For this review, take the finished solid that the model builds, in its own axes (mm). A direction names the side the tool comes from. Give positions to 0.01 mm unless a question says otherwise; leave off trailing zeros. Order: outer loops, then holes, each group sorted by start corner. A loop starts at its lowest first (then second) coordinate and runs counter-clockwise, first axis right, second up.
from build123d import *

# Parameters (mm, degrees)
SKETCH_1_R      = 2.5
EXTRUDE_1_DEPTH = 3
THICKEN_1_DEPTH = 2
FILLET_6_R      = 4


# Read off the part's stored shape, not the designer's step: 加厚1
with BuildPart() as part:
    # 草图1 → 凸台-拉伸1 (new body)
    with BuildSketch(Plane.XZ):
        with BuildLine():
            Line((-97.488460856, 0), (-69, 0))
            ThreePointArc((-69, 0), (-65, -4), (-61, 0))
            Line((-61, 0), (61, 0))
            ThreePointArc((61, 0), (65, -4), (69, 0))
            Line((69, 0), (97.488460856, 0))
            ThreePointArc((97.488460856, 0), (79.00867922, -47.979553361), (38.781438859, -80))
            Line((38.781438859, -80), (15.564382416, -80))
            ThreePointArc((15.564382416, -80), (0, -70.5), (-15.564382416, -80))
            Line((-15.564382416, -80), (-38.781438859, -80))
            ThreePointArc((-38.781438859, -80), (-79.00867922, -47.979553361), (-97.488460856, 0))
        make_face()
        with Locations(Location((75, -15, 0), (0, 0, 270))):
            Circle(SKETCH_1_R, mode=Mode.SUBTRACT)
    extrude(amount=EXTRUDE_1_DEPTH)

    # 加厚1 outline → 加厚1 (add)
    with BuildSketch(Plane(origin=(0, 0, 0), x_dir=(1, 0, 0), z_dir=(0, 1, 0))):
        with BuildLine():
            ThreePointArc((16.853782958, 77.8), (0, 68.3), (-16.853782958, 77.8))
            Line((-16.853782958, 77.8), (-38.324926614, 77.8))
            ThreePointArc((-38.324926614, 77.8), (-76.642398339, 47.476802076), (-95.019997895, 2.2))
            Line((-95.019997895, 2.2), (-70.796550698, 2.2))
            ThreePointArc((-70.796550698, 2.2), (-65, 6.2), (-59.203449302, 2.2))
            Line((-59.203449302, 2.2), (59.203449302, 2.2))
            ThreePointArc((59.203449302, 2.2), (65, 6.2), (70.796550698, 2.2))
            Line((70.796550698, 2.2), (95.019997895, 2.2))
            ThreePointArc((95.019997895, 2.2), (76.642398339, 47.476802076), (38.324926614, 77.8))
            Line((38.324926614, 77.8), (16.853782958, 77.8))
        make_face()
        with BuildLine():
            Line((-38.115613599, 76.8), (-17.408331339, 76.8))
            ThreePointArc((-17.408331339, 76.8), (0, 67.3), (17.408331339, 76.8))
            Line((17.408331339, 76.8), (38.115613599, 76.8))
            ThreePointArc((38.115613599, 76.8), (75.562692375, 47.247877874), (93.876514635, 3.2))
            Line((93.876514635, 3.2), (71.449806199, 3.2))
            ThreePointArc((71.449806199, 3.2), (65, 7.2), (58.550193801, 3.2))
            Line((58.550193801, 3.2), (-58.550193801, 3.2))
            ThreePointArc((-58.550193801, 3.2), (-65, 7.2), (-71.449806199, 3.2))
            Line((-71.449806199, 3.2), (-93.876514635, 3.2))
            ThreePointArc((-93.876514635, 3.2), (-75.562692375, 47.247877874), (-38.115613599, 76.8))
        make_face(mode=Mode.SUBTRACT)
    extrude(amount=THICKEN_1_DEPTH)

    # 圆角6
    fillet_6_edges = [part.edges().sort_by_distance(p)[0] for p in [
        (-38.781438859, -1.5, -80),
        (-15.564382416, -1.5, -80),
        (15.564382416, -1.5, -80),
        (38.781438859, -1.5, -80),
        (-38.324926614, 1, -77.8),
        (-16.853782958, 1, -77.8),
        (16.853782958, 1, -77.8),
    ]]
    fillet(fillet_6_edges, radius=FILLET_6_R)


solid = part.part
1) Draft analysis for pull direction X (two halves, no side actions). For faces 1 (the face through (-65, -1, -4)), 2 (the face through (-78.83, -1.48, -48.22)), 3 (the face through (77, 1, -47)), 4 (the face through (64.9, 1, -6.2)), state which applies: +X half, -X half, draft (parallel to the pull), parting line (faces both ways), or undercut.
Answer sheet:
face 1: undercut
face 2: -X half
face 3: +X half
face 4: undercut
2) Clearance check with flat-ended pins moving along their axes: pin 1 (1.6 mm diameter, centred on x = -31, y = 1.5, fed in from +Z); pin 2 (2 mm diameter, centred on x = 29.5, y = 1.5, fed in from -Z); pin 3 (1 mm diameter, centred on y = 0, z = -19.5, fed in from +X). State where each tip first meets the part, or that it passes through.
Answer sheet:
pin 1: stops at z = -2.2
pin 2: stops at z = -77.8
pin 3: stops at x = 93.61
3) Tool access review of faces 5 (the face through (1, -3, -31)), 6 (the face through (75.153, 0.986, -47.785)), 7 (the face through (0.26, 0.99, -68.3)), 8 (the face through (-65.1, 1, -6.2)), 9 (the face through (-76.49, 0.99, -47.68)): name each direction out of +Z, -Z, +X, -X, +Y, -Y from which nothing blocks a thin tool from reaching the whole face with its end or side.
Answer sheet:
face 5: +Z, -Z, +X, -X, -Y
face 6: +Y
face 7: -Z, +Y
face 8: +Z, +Y
face 9: -Z, -X, +Y
4) We need section D-D on x = 28. Give the boundary of the cut face in (y, z), then the cut area to 3 significant figures.
Answer sheet:
outline: (-3, -80) - (0, -80) - (0, -77.8) - (2, -77.8) - (2, -76.8) - (0, -76.8) - (0, -3.2) - (2, -3.2) - (2, -2.2) - (0, -2.2) - (0, 0) - (-3, 0) - close
area: 244 mm2
5) We need section C-C on z = -15. Give the boundary of the cut face in (x, y).
Answer sheet:
outline: (-94.76, -3) - (72.5, -3) - (72.5, 0) - (-91.44, 0) - (-91.44, 2) - (-92.48, 2) - (-92.48, 0) - (-94.76, 0) - close; (77.5, -3) - (94.76, -3) - (94.76, 0) - (92.48, 0) - (92.48, 2) - (91.44, 2) - (91.44, 0) - (77.5, 0) - close
6) We need section B-B on x = 75. Give the boundary of the cut face in (y, z), then the cut area to 3 significant figures.
Answer sheet:
outline: (-3, -53.08) - (0, -53.08) - (0, -49.6) - (2, -49.6) - (2, -47.98) - (0, -47.98) - (0, -17.5) - (-3, -17.5) - close; (-3, -12.5) - (0, -12.5) - (0, -3.2) - (2, -3.2) - (2, -2.2) - (0, -2.2) - (0, 0) - (-3, 0) - close
area: 149 mm2
7) We need section A-A on y = -1.6. Give the boundary of the cut face in (x, z).
Answer sheet:
outline: (-97.49, 0) arc R98 ccw to (-39.56, -79.66) arc R4 ccw to (-37.95, -80) - (-17.84, -80) arc R4 ccw to (-14.52, -78.23) arc R17.5 cw to (14.52, -78.23) arc R4 ccw to (17.84, -80) - (37.95, -80) arc R4 ccw to (39.56, -79.66) arc R98 ccw to (97.49, 0) - (69, 0) arc R4 cw to (61, 0) - (-61, 0) arc R4 cw to (-69, 0) - close; hole circle Ø5 at (75, -15)
8) To check wall thickness, follow line 1 (Z direction, x = -28, y = 0.25); line 2 (Y direction, x = 14, z = -65); line 3 (Z direction, x = 1, y = -1.2). State the ranges of each line that lie inside material, in increasing order.
Answer sheet:
line 1: z = -77.8 to -76.8, -3.2 to -2.2
line 2: y = -3 to 0
line 3: z = -70.53 to 0
